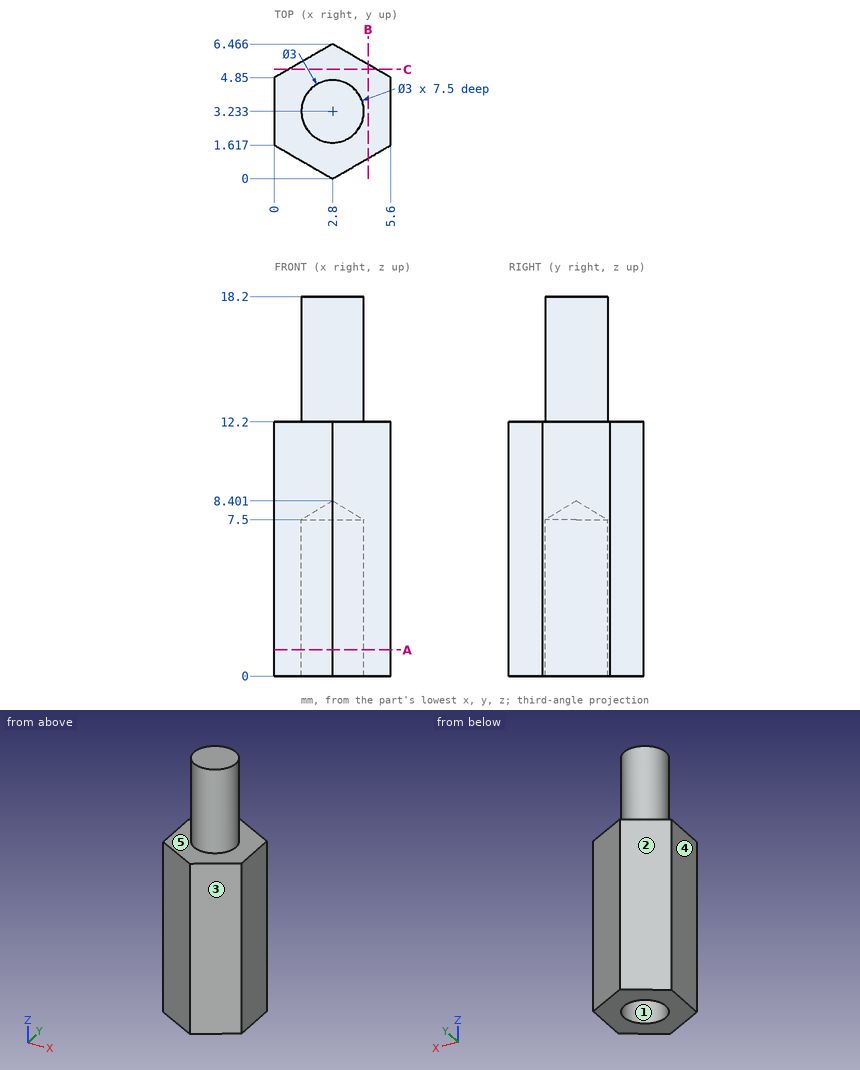
Input: dimensioned drawing with shaded views. Units: mm. Origin: part minimum x, y, z. A direction names the side the tool comes from. Coordinates: 2 decimals unless noted, no trailing zeros. Write each loop counter-clockwise with the first axis right and the second up, starting at its lowest first coordinate (ties: lowest second). Pieces come first, ordered by that corner, then holes. Notation, with made-up numbers: (37, 74) -> (66, 74) arc R11 ccw to (66, 79) -> close; hole circle Ø6 at (-5.5, -4). An arc over 180 degrees is marked (long way). Return JSON: item names as keys, results as strings. Group by question number.
1) Section query A-A, the plane z = 1.25. Return loops of the section in (x, y), plus the area to 3 significant figures.
2) Mould query, pull axis Y, two halves, no side actions, for the marked faces 1, 2 and 3. Classes: +Y half, -Y half, draft (parallel to the pull), parting line (faces both ways), or undercut.
3) Ray query, line 1 along Z through (x, y) = (4.9, 1.25); line 2 along Y through (x, z) = (2.75, 4.75) (1 decimal); line 3 along X through (y, z) = (2.25, 1) (1 decimal). Return the intervals inside material, ascending.
4) Contact query for flat-ended pins moving along their axis: P1, Ø1.5, axis at x = 1.5, z = 9.5, coming from the +Y side; P2, Ø1.8, axis at x = 2.8, y = 3.23, coming from the -Z side. Output: stop coordinate, or through.
5) Section query C-C, the plane y = 5.25. Return loops of the section in (x, z), plus the area to 3 significant figures.
6) Section query B-B, the plane x = 4.5. Return loops of the section in (y, z) (1 decimal).
7) Set-up query: the marked faces 4 and 5. Return all of +Z, -Z, +X, -X, +Y, -Y with unobstructed straight access to the full face (end or side cutting, diameter ignored); none if empty.
From the geometry:
{
 "1": {"outline": "(0, 1.62) -> (2.8, 0) -> (5.6, 1.62) -> (5.6, 4.85) -> (2.8, 6.47) -> (0, 4.85) -> close; hole circle Ø3 at (2.8, 3.23)", "area": "20.1 mm²"},
 "2": {"face 1": "undercut", "face 2": "+Y half", "face 3": "-Y half"},
 "3": {"line 1": "0 to 12.2", "line 2": "0 to 1.7, 4.7 to 6.4", "line 3": "0 to 1.7, 3.9 to 5.6"},
 "4": {"P1": "y = 6.15", "P2": "z = 7.86"},
 "5": {"outline": "(0.69, 0) -> (4.91, 0) -> (4.91, 12.2) -> (0.69, 12.2) -> close", "area": "51.4 mm²"},
 "6": {"outline": "(1, 0) -> (5.5, 0) -> (5.5, 12.2) -> (1, 12.2) -> close"},
 "7": {"face 4": "+Z, -Z, -X, +Y, -Y", "face 5": "+Z"}
}
